from build123d import *
from build123d.topology import SkipClean

# Parameters (mm, degrees)
EXTRUDE_1_DEPTH           = 20
SKETCH_3_R                = 5.5
CUT_EXTRUDE_2_DEPTH       = 10
SKETCH_9_R                = 6.25
CUT_EXTRUDE_6_DEPTH       = 1
SKETCH_11_W               = 20
SKETCH_11_H               = 5
EXTRUDE_4_DEPTH           = 10
CUT_EXTRUDE_8_REACH       = 78.472
SKETCH_12_R               = 1.5
SKETCH_13_R               = 3
CUT_EXTRUDE_9_DEPTH       = 2.5
SKETCH_14_R               = 10
SKETCH_14_R_2             = 5.5
EXTRUDE_5_DEPTH           = 6
CUT_EXTRUDE_START         = -1
SKETCH_6_R                = 6.25
CUT_EXTRUDE_10_DEPTH      = 1
SKETCH_15_W               = 20
SKETCH_15_H               = 5
EXTRUDE_6_DEPTH           = 5
SKETCH_16_W               = 17
SKETCH_16_H               = 3
EXTRUDE_7_DEPTH           = 15
CUT_EXTRUDE_11_DEPTH      = 70.961190435
CUT_EXTRUDE_11_DEPTH_BACK = 70.961190435
EXTRUDE_START             = -5
SKETCH_3D_3_R             = 1.5
EXTRUDE_8_DEPTH           = 5
CUT_EXTRUDE_12_DEPTH      = 2.5
FILLET_1_R                = 2
CUT_EXTRUDE_14_DEPTH      = 76.06644022
SKETCH_21_W               = 6.587713241
SKETCH_21_H               = 4.5
EXTRUDE_9_DEPTH           = 15
SKETCH_23_W               = 25
SKETCH_23_H               = 20
CUT_EXTRUDE_16_DEPTH      = 5
CUT_EXTRUDE_17_DEPTH      = 10
SKETCH_25_W               = 10
SKETCH_25_H               = 20
EXTRUDE_10_DEPTH          = 3
SKETCH_26_R               = 1.5
CUT_EXTRUDE_18_DEPTH      = 71.326165394
SKETCH_27_R               = 1.5
CUT_EXTRUDE_19_DEPTH      = 71.326165394


with BuildPart() as part:
    # 草图1 → 凸台-拉伸1 (new body)
    with BuildSketch(Plane.XY):
        Polygon((-63.866818046, 22.947717095), (-23.866818046, 22.947717095), (-23.866818046, -19.052282905), (-33.866818046, -19.052282905), (-33.866818046, 14.947717095), (-63.866818046, 14.947717095), align=None)
    extrude(amount=EXTRUDE_1_DEPTH)

    # 草图3 → 切除-拉伸2 (cut)
    with BuildSketch(Plane(origin=(0, 22.947717095, 0), x_dir=(-1, 0, 0), z_dir=(0, 1, 0))):
        with Locations((50.866818046, 10)):
            Circle(SKETCH_3_R)
    extrude(amount=-CUT_EXTRUDE_2_DEPTH, mode=Mode.SUBTRACT)

    # 草图9 → 切除-拉伸6 (cut)
    with BuildSketch(Plane(origin=(0, 22.947717095, 0), x_dir=(1, 0, 0), z_dir=(0, 1, 0))):
        with Locations(Location((-50.866818046, -10, 0), (0, 0, 180))):
            Circle(SKETCH_9_R)
    extrude(amount=-CUT_EXTRUDE_6_DEPTH, mode=Mode.SUBTRACT)

    # 草图11 → 凸台-拉伸4 (add)
    with BuildSketch(Plane(origin=(-23.866818046, 0, 0), x_dir=(0, 0, -1), z_dir=(1, 0, 0))):
        with Locations((-10, -16.552282905)):
            Rectangle(SKETCH_11_W, SKETCH_11_H)
    extrude(amount=EXTRUDE_4_DEPTH)

    # 草图12 → 切除-拉伸8 (cut, up to next)
    with BuildSketch(Plane(origin=(0, -14.052282905, 0), x_dir=(-1, 0, 0), z_dir=(0, 1, 0)), mode=Mode.PRIVATE) as cut_extrude_8_sk1:
        with Locations((18.866818046, 5)):
            Circle(SKETCH_12_R)
    cut_extrude_8_tool1 = extrude(cut_extrude_8_sk1.sketch, amount=-CUT_EXTRUDE_8_REACH, mode=Mode.PRIVATE) & part.part
    # 草图12 → 切除-拉伸8 (cut, up to next)
    with BuildSketch(Plane(origin=(0, -14.052282905, 0), x_dir=(-1, 0, 0), z_dir=(0, 1, 0)), mode=Mode.PRIVATE) as cut_extrude_8_sk2:
        with Locations((18.866818046, 15)):
            Circle(SKETCH_12_R)
    cut_extrude_8_tool2 = extrude(cut_extrude_8_sk2.sketch, amount=-CUT_EXTRUDE_8_REACH, mode=Mode.PRIVATE) & part.part
    add(cut_extrude_8_tool1.solids().sort_by_distance((-18.866818, -14.052283, 5))[0], mode=Mode.SUBTRACT)
    add(cut_extrude_8_tool2.solids().sort_by_distance((-18.866818, -14.052283, 15))[0], mode=Mode.SUBTRACT)

    # 草图13 → 切除-拉伸9 (cut)
    with BuildSketch(Plane.XZ.offset(19.052282905)):
        with Locations(Location((-18.866818046, 15, 0), (0, 0, 270))):
            Circle(SKETCH_13_R)
        with Locations(Location((-18.866818046, 5, 0), (0, 0, 270))):
            Circle(SKETCH_13_R)
    extrude(amount=-CUT_EXTRUDE_9_DEPTH, mode=Mode.SUBTRACT)

    # 草图14 → 凸台-拉伸5 (add)
    with SkipClean():  # the faces are left unmerged after this step: merging them gives an invalid solid
        with BuildSketch(Plane.XZ.offset(-14.947717095)):
            with Locations(Location((-50.866818046, 10, 0), (0, 0, 270))):
                Circle(SKETCH_14_R)
            with Locations(Location((-50.866818046, 10, 0), (0, 0, 180))):
                Circle(SKETCH_14_R_2, mode=Mode.SUBTRACT)
        extrude(amount=EXTRUDE_5_DEPTH)

    # 草图6 → 切除-拉伸10 (cut)
    with BuildSketch(Plane.XZ.offset(-8.947717095).offset(CUT_EXTRUDE_START)):
        with Locations(Location((-50.866818046, 10, 0), (0, 0, 180))):
            Circle(SKETCH_6_R)
    extrude(amount=CUT_EXTRUDE_10_DEPTH, mode=Mode.SUBTRACT)

    # 草图15 → 凸台-拉伸6 (add)
    with BuildSketch(Plane(origin=(-13.866818046, 0, 0), x_dir=(0, 0, -1), z_dir=(1, 0, 0))):
        with Locations((-10, -16.552282905)):
            Rectangle(SKETCH_15_W, SKETCH_15_H)
    extrude(amount=EXTRUDE_6_DEPTH)

    # 草图16 → 凸台-拉伸7 (add)
    with BuildSketch(Plane.XZ.offset(-14.947717095)):
        with Locations((-42.366818046, 18.5)):
            Rectangle(SKETCH_16_W, SKETCH_16_H)
        with Locations((-42.366818046, 1.5)):
            Rectangle(SKETCH_16_W, SKETCH_16_H)
    extrude(amount=EXTRUDE_7_DEPTH)

    # 草图17 → 切除-拉伸11 (cut, two sides: drawn at the far end of the back side and taken through both)
    with BuildSketch(Plane(origin=(0, 0, 17), x_dir=(-1, 0, 0), z_dir=(0, 0, -1)).offset(-CUT_EXTRUDE_11_DEPTH_BACK)):
        Polygon((50.866818046, 8.947717095), (43.725389617, 8.947717095), (33.866818046, -0.052282905), (50.866818046, -0.052282905), align=None)
    extrude(amount=CUT_EXTRUDE_11_DEPTH + CUT_EXTRUDE_11_DEPTH_BACK, mode=Mode.SUBTRACT)

    # Sketch 3D_3 → 凸台-拉伸8 (add)
    with BuildSketch(Plane(origin=(-23.866818046, -6.052282905, 20), x_dir=(0.447213595499958, 0, -0.894427190999916), z_dir=(0, -1, 0)).offset(EXTRUDE_START)):
        Polygon((0, 0), (4.472135955, 8.94427191), (22.360679775, 0), (17.88854382, -8.94427191), align=None)
        with Locations(Location((6.708203932, 2.236067977, 0), (0, 0, 243.434948823))):
            Circle(SKETCH_3D_3_R, mode=Mode.SUBTRACT)
        with Locations(Location((15.652475842, -2.236067977, 0), (0, 0, 243.434948823))):
            Circle(SKETCH_3D_3_R, mode=Mode.SUBTRACT)
    extrude(amount=EXTRUDE_8_DEPTH)

    # 草图18 → 切除-拉伸12 (cut)
    with BuildSketch(Plane(origin=(0, -1.052282905, 0), x_dir=(-1, 0, 0), z_dir=(0, 1, 0))):
        Polygon((15.691391565, 15), (17.279104805, 12.25), (20.454531286, 12.25), (22.042244526, 15), (20.454531286, 17.75), (17.279104805, 17.75), align=None)
        Polygon((15.691391565, 5), (17.279104805, 2.25), (20.454531286, 2.25), (22.042244526, 5), (20.454531286, 7.75), (17.279104805, 7.75), align=None)
    extrude(amount=-CUT_EXTRUDE_12_DEPTH, mode=Mode.SUBTRACT)

    # 圆角1
    # the kernel refuses this fillet: 2 mm, written as the material it adds along each edge
    with BuildSketch(Plane(origin=(-23.866818046, -1.052282905, 0), x_dir=(0, 1, 0), z_dir=(0, 0, 1))) as fillet_1_piece_1_section:
        with BuildLine():
            CenterArc((FILLET_1_R, -FILLET_1_R), FILLET_1_R, 90, 90)
            Line((0, -FILLET_1_R), (0, 0))
            Line((0, 0), (FILLET_1_R, 0))
        make_face()
    fillet_1_piece_1 = extrude(amount=20, mode=Mode.PRIVATE)
    fillet_1_piece_1 = split(fillet_1_piece_1, bisect_by=Plane(origin=(-20.802583542, -0.671658343, 2.852844192), z_dir=(-0.8660254037844387, 0, -0.5000000000000001)), keep=Keep.TOP, mode=Mode.PRIVATE)
    fillet_1_piece_1 = split(fillet_1_piece_1, bisect_by=Plane(origin=(-23.907001975, -0.671658343, 1.770145354), z_dir=(0.8660254037844387, 0, -0.5000000000000003)), keep=Keep.TOP, mode=Mode.PRIVATE)
    add(fillet_1_piece_1)
    with BuildSketch(Plane(origin=(-23.866818046, -1.052282905, 0), x_dir=(0, 1, 0), z_dir=(0, 0, 1))) as fillet_1_piece_2_section:
        with BuildLine():
            CenterArc((FILLET_1_R, -FILLET_1_R), FILLET_1_R, 90, 90)
            Line((0, -FILLET_1_R), (0, 0))
            Line((0, 0), (FILLET_1_R, 0))
        make_face()
    fillet_1_piece_2 = extrude(amount=20, mode=Mode.PRIVATE)
    fillet_1_piece_2 = split(fillet_1_piece_2, bisect_by=Plane(origin=(-22.4188867, -0.519681884, 5.652363381), z_dir=(-0.8660254037844387, 0, -0.5000000000000001)), keep=Keep.TOP, mode=Mode.PRIVATE)
    fillet_1_piece_2 = split(fillet_1_piece_2, bisect_by=Plane(origin=(-22.4188867, -0.519681884, 4.347636619), z_dir=(-0.8660254037844387, 0, 0.5000000000000003)), keep=Keep.TOP, mode=Mode.PRIVATE)
    add(fillet_1_piece_2)
    with BuildSketch(Plane(origin=(-23.866818046, -1.052282905, 0), x_dir=(0, 1, 0), z_dir=(0, 0, 1))) as fillet_1_piece_3_section:
        with BuildLine():
            CenterArc((FILLET_1_R, -FILLET_1_R), FILLET_1_R, 90, 90)
            Line((0, -FILLET_1_R), (0, 0))
            Line((0, 0), (FILLET_1_R, 0))
        make_face()
    fillet_1_piece_3 = extrude(amount=20, mode=Mode.PRIVATE)
    fillet_1_piece_3 = split(fillet_1_piece_3, bisect_by=Plane(origin=(-24.519856268, -0.671658343, 9.291349419), z_dir=(0.8660254037844387, 0, 0.5000000000000001)), keep=Keep.TOP, mode=Mode.PRIVATE)
    fillet_1_piece_3 = split(fillet_1_piece_3, bisect_by=Plane(origin=(-20.189729249, -0.671658343, 8.208650581), z_dir=(-0.8660254037844387, 0, 0.5000000000000003)), keep=Keep.TOP, mode=Mode.PRIVATE)
    fillet_1_piece_3 = split(fillet_1_piece_3, bisect_by=Plane(origin=(-20.189729249, -0.671658343, 11.791349419), z_dir=(-0.8660254037844387, 0, -0.5)), keep=Keep.TOP, mode=Mode.PRIVATE)
    fillet_1_piece_3 = split(fillet_1_piece_3, bisect_by=Plane(origin=(-24.519856268, -0.671658343, 10.708650581), z_dir=(0.8660254037844384, 0, -0.5000000000000004)), keep=Keep.TOP, mode=Mode.PRIVATE)
    add(fillet_1_piece_3)
    with BuildSketch(Plane(origin=(-23.866818046, -1.052282905, 0), x_dir=(0, 1, 0), z_dir=(0, 0, 1))) as fillet_1_piece_4_section:
        with BuildLine():
            CenterArc((FILLET_1_R, -FILLET_1_R), FILLET_1_R, 90, 90)
            Line((0, -FILLET_1_R), (0, 0))
            Line((0, 0), (FILLET_1_R, 0))
        make_face()
    fillet_1_piece_4 = extrude(amount=20, mode=Mode.PRIVATE)
    fillet_1_piece_4 = split(fillet_1_piece_4, bisect_by=Plane(origin=(-22.4188867, -0.519681884, 15.652363381), z_dir=(-0.8660254037844387, 0, -0.5)), keep=Keep.TOP, mode=Mode.PRIVATE)
    fillet_1_piece_4 = split(fillet_1_piece_4, bisect_by=Plane(origin=(-22.4188867, -0.519681884, 14.347636619), z_dir=(-0.8660254037844384, 0, 0.5000000000000004)), keep=Keep.TOP, mode=Mode.PRIVATE)
    add(fillet_1_piece_4)
    with BuildSketch(Plane(origin=(-23.866818046, -1.052282905, 0), x_dir=(0, 1, 0), z_dir=(0, 0, 1))) as fillet_1_piece_5_section:
        with BuildLine():
            CenterArc((FILLET_1_R, -FILLET_1_R), FILLET_1_R, 90, 90)
            Line((0, -FILLET_1_R), (0, 0))
            Line((0, 0), (FILLET_1_R, 0))
        make_face()
    fillet_1_piece_5 = extrude(amount=20, mode=Mode.PRIVATE)
    fillet_1_piece_5 = split(fillet_1_piece_5, bisect_by=Plane(origin=(-23.907001975, -0.671658343, 18.229854646), z_dir=(0.8660254037844387, 0, 0.5)), keep=Keep.TOP, mode=Mode.PRIVATE)
    fillet_1_piece_5 = split(fillet_1_piece_5, bisect_by=Plane(origin=(-20.802583542, -0.671658343, 17.147155808), z_dir=(-0.8660254037844384, 0, 0.5000000000000004)), keep=Keep.TOP, mode=Mode.PRIVATE)
    add(fillet_1_piece_5)

    # 草图20 → 切除-拉伸14 (cut, through all)
    with SkipClean():  # the faces are left unmerged after this step: merging them gives an invalid solid
        with BuildSketch(Plane.XZ.offset(-14.947717095)):
            with BuildLine():
                Line((-63.866818046, 20), (-50.866818046, 20))
                ThreePointArc((-50.866818046, 20), (-60.866818046, 10), (-50.866818046, 0))
                Line((-50.866818046, 0), (-63.866818046, 0))
                Line((-63.866818046, 0), (-63.866818046, 20))
            make_face()
        extrude(amount=-CUT_EXTRUDE_14_DEPTH, mode=Mode.SUBTRACT)
    add(part.part.scale(1), mode=Mode.REPLACE)  # the faces are merged on a copy

    # 草图21 → 凸台-拉伸9 (add)
    with BuildSketch(Plane(origin=(0, -1.052282905, 0), x_dir=(1, 0, 0), z_dir=(0, 1, 0))):
        with Locations((-20.572961426, -10)):
            Rectangle(SKETCH_21_W, SKETCH_21_H)
    extrude(amount=EXTRUDE_9_DEPTH)

    # 草图23 → 切除-拉伸16 (cut)
    with BuildSketch(Plane.XZ.offset(19.052282905)):
        with Locations((-21.366818046, 10)):
            Rectangle(SKETCH_23_W, SKETCH_23_H)
    extrude(amount=-CUT_EXTRUDE_16_DEPTH, mode=Mode.SUBTRACT)

    # 草图24 → 切除-拉伸17 (cut)
    with BuildSketch(Plane.XY.offset(12.25)):
        Polygon((-23.866818046, 13.947717095), (-17.279104805, -1.052282905), (-17.279104805, 13.947717095), align=None)
    extrude(amount=-CUT_EXTRUDE_17_DEPTH, mode=Mode.SUBTRACT)

    # 草图25 → 凸台-拉伸10 (add)
    with BuildSketch(Plane.XZ.offset(6.052282905)):
        with Locations((-18.866818046, 10)):
            Rectangle(SKETCH_25_W, SKETCH_25_H)
    extrude(amount=EXTRUDE_10_DEPTH)

    # 草图26 → 切除-拉伸18 (cut, through all)
    with BuildSketch(Plane(origin=(0, -6.052282905, 0), x_dir=(1, 0, 0), z_dir=(0, 1, 0))):
        with Locations(Location((-18.866818046, -15, 0), (0, 0, 270))):
            Circle(SKETCH_26_R)
    extrude(amount=-CUT_EXTRUDE_18_DEPTH, mode=Mode.SUBTRACT)

    # 草图27 → 切除-拉伸19 (cut, through all)
    with BuildSketch(Plane(origin=(0, -6.052282905, 0), x_dir=(1, 0, 0), z_dir=(0, 1, 0))):
        with Locations(Location((-18.866818046, -5, 0), (0, 0, 270))):
            Circle(SKETCH_27_R)
    extrude(amount=-CUT_EXTRUDE_19_DEPTH, mode=Mode.SUBTRACT)


solid = part.part
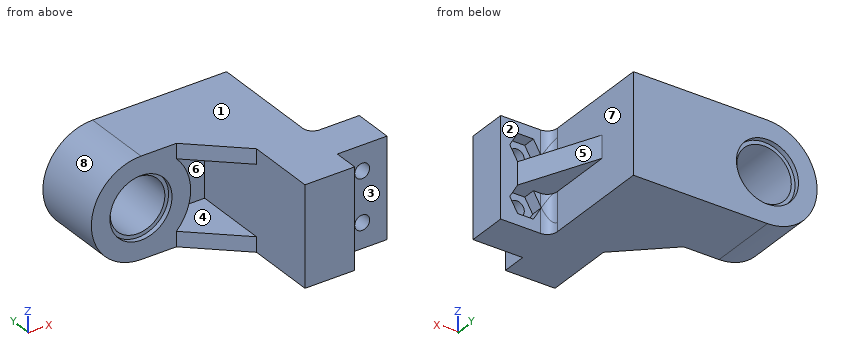
Verification items for the finished model (mm, model axes). Face numbers are marked on the shaded views. A direction names the side the tool comes from. Give positions to 0.01 mm unless a question says otherwise; leave off trailing zeros. Order: outer loops, then holes, each group sorted by start corner. A loop starts at its lowest first (then second) coordinate and runs counter-clockwise, first axis right, second up. Notation, with made-up numbers: M -39,31 L -1,31 A24 cw -1,66 Z; hole C 51,23.5 d5. An arc over 180 degrees is marked long. Use one line per item in the form item = value. Start each with the question number.
Q1. Scan lines: line 1 along Z through (x, y) = (-35, 7); line 2 along X through (y, z) = (9.6, 10); line 3 along X through (y, z) = (-7.95, 15). Record each from-to range of solid material in increasing order. Write a range as [from, to].
Q2. Mould release check, pull along Z, two halves, no side actions. Record for the marked faces 6, 7 and 8: +Z half, -Z half, draft (parallel to the pull), parting line (faces both ways), or undercut.
Q3. Go/stop test with flat-tipped pins: pin 1 Ø5 at (x, z) = (-18.87, 5) entering from -Y; pin 2 Ø10 at (x, z) = (-49, 6) entering from -Y; pin 3 Ø1.8 at (x, z) = (-18.87, 15) entering from +Y; pin 4 Ø8 at (y, z) = (-6, 6.5) entering from -X. Record where each tip stops, or that it passes through.
Q4. Section check C-C (y = -7.5). Enter the section's corners in (x, z), then the cut area to 3 significant figures.
Q5. Section check B-B (y = 17.5). Enter the section's corners in (x, z).
Q6. Section check A-A (z = 10). Enter the section's corners in (x, y).
Q7. Access from +Z, -Z, +X, -X, +Y, -Y to the whole of each face (thin tool, end or side, straight path). Record for the marked faces 1, 2, 3, 4 and 5.
Evaluation:
q1.line_1 = [0, 3], [17, 20]
q1.line_2 = [-60.87, -57.12], [-44.62, -40.87], [-33.87, -21.96]
q1.line_3 = [-33.87, -20.37], [-17.37, -13.87]
q2.face_6 = undercut
q2.face_7 = draft
q2.face_8 = parting line
q3.pin_1 = -9.05
q3.pin_2 = 8.95
q3.pin_3 = through
q3.pin_4 = -33.87
q4.outline = M -33.87,0 L -13.87,0 L -13.87,20 L -33.87,20 Z; hole C -18.87,5 d3; hole C -18.87,15 d3
q4.area = 386 mm2
q5.outline = M -50.87,0 L -23.87,0 L -23.87,20 L -50.87,20 A10 ccw Z; hole C -50.87,10 d11
q6.outline = M -60.87,8.95 L -57.12,8.95 L -57.12,9.95 L -56.37,9.95 L -56.37,21.95 L -57.12,21.95 L -57.12,22.95 L -60.87,22.95 Z; M -45.37,9.95 L -44.62,9.95 L -44.62,8.95 L -40.87,8.95 L -40.87,14.95 L -33.87,14.95 L -33.87,-14.05 L -23.87,-14.05 L -23.87,-9.05 L -13.87,-9.05 L -13.87,-1.05 L -17.28,-1.05 L -23.87,13.95 L -23.87,22.95 L -44.62,22.95 L -44.62,21.95 L -45.37,21.95 Z
q7.face_1 = +Z, +X, -X, +Y, -Y
q7.face_2 = +X, +Y
q7.face_3 = +Z, -Z, +X, -Y
q7.face_4 = -Y
q7.face_5 = +Z, -Z, +X, +Y
